from build123d import *

# Parameters (mm, degrees)
F0_R     = 11.75
F0_R_2   = 11.25
F1_DEPTH = 10
F2_R     = 15.213548
F2_R_2   = 11.75
F3_DEPTH = 10
F4_SIZE  = 1
F5_SIZE  = 1


with BuildPart() as f1:
    # F0 (on Top) → F1 (new body)
    with BuildSketch(Plane.XY):
        Circle(F0_R)
        Circle(F0_R_2, mode=Mode.SUBTRACT)
    extrude(amount=-F1_DEPTH)

    # F2 (on Top) → F3 (join)
    with BuildSketch(Plane.XY):
        Circle(F2_R)
        Circle(F2_R_2, mode=Mode.SUBTRACT)
    extrude(amount=-F3_DEPTH)

    # F4
    f4_edges = [f1.edges().sort_by_distance(p)[0] for p in [
        (-11.25, 0, 0),
    ]]
    chamfer(f4_edges, length=F4_SIZE)

    # F5
    f5_edges = [f1.edges().sort_by_distance(p)[0] for p in [
        (-11.25, 0, -10),
    ]]
    chamfer(f5_edges, length=F5_SIZE)


solid = f1.part
For this review, take the finished solid that the model builds, in its own axes (mm). Round coordinates to 2 decimals unless told otherwise and drop trailing zeros. Write each loop counter-clockwise with the first axis right and the second up, starting at its lowest first coordinate (ties: lowest second). Pieces come first, ordered by that corner, then holes. Notation, with made-up numbers: (47.25, 0) - (79.25, 0) arc R18 ccw to (79.25, 28) - close; hole circle Ø4 at (68.5, -1). An arc over 180 degrees is marked (long way). Use a Markdown table: item, result.
Q1. We need section A-A (x = 0). Give the boundary of the cut face in (y, z).
Derived:
| item | result |
|---|---|
| outline | (-15.21, -10) - (-12.25, -10) - (-11.25, -9) - (-11.25, -1) - (-12.25, 0) - (-15.21, 0) - close; (11.25, -9) - (12.25, -10) - (15.21, -10) - (15.21, 0) - (12.25, 0) - (11.25, -1) - close |
Q2. The part is to be moulded in two halves that separate along Y. For faces 1 (the cylindrical face through (5.19, -9.98, -4.94)), 2 (the flat face through (1.1, 12.5, -10)), 3 (the cylindrical face through (-11.213, 10.282, -4.93)), say which applies: pulls with the +Y half, pulls with the -Y half, needs draft (parallel to the pull), parting line crosses it, or undercut.
Derived:
| item | result |
|---|---|
| face 1 | undercut |
| face 2 | needs draft |
| face 3 | parting line crosses it |
Q3. We need section D-D (z = -8.25). Give the boundary of the cut face in (x, y).
Derived:
| item | result |
|---|---|
| outline | circle Ø30.43 at (0, 0); hole circle Ø22.5 at (0, 0) |
Q4. Clearance check with flat-ended pins moving along their axes: pin 1 (3 mm diameter, centred on x = 10.5, y = 5.5, fed in from -Z); pin 2 (4 mm diameter, centred on x = 12, z = -1, fed in from -Y); pin 3 (2 mm diameter, centred on x = -10.5, y = 0, fed in from -Z). State where each tip first meets the part, or that it passes through.
Derived:
| item | result |
|---|---|
| pin 1 | stops at z = -10 |
| pin 2 | stops at y = -11.47 |
| pin 3 | stops at z = -9.25 |
Q5. We need section C-C (z = -0.5). Give the boundary of the cut face in (x, y).
Derived:
| item | result |
|---|---|
| outline | circle Ø30.43 at (0, 0); hole circle Ø23.5 at (0, 0) |
Q6. Wall thickness on line 1 along Y through (x, z) = (0, -5); line 2 along X through (y, z) = (4.5, -7.5); line 3 along Y through (x, z) = (-3.5, -8.25): over which ranges is each line inside the solid? List them lowest first.
Derived:
| item | result |
|---|---|
| line 1 | y = -15.21 to -11.25, 11.25 to 15.21 |
| line 2 | x = -14.53 to -10.31, 10.31 to 14.53 |
| line 3 | y = -14.81 to -10.69, 10.69 to 14.81 |
